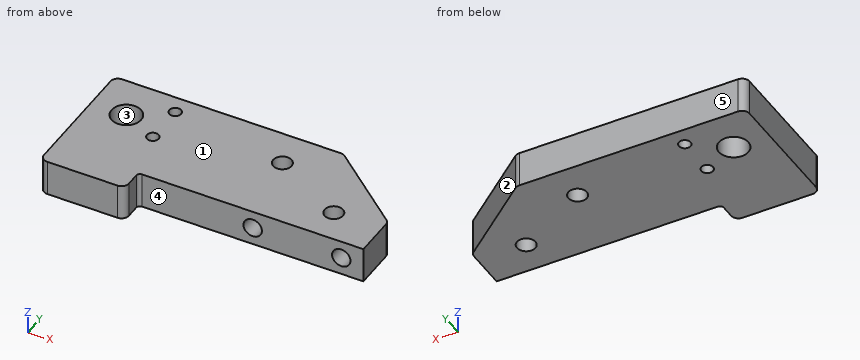
```python
from build123d import *

# Parameters (mm, degrees)
BOSS_EXTRUDE1_DEPTH             = 4.826
M3X0_5_TAPPED_HOLE1_D           = 2.5
TAP_DRILL_FOR_M3X0_5_TAP1_D     = 2.5
TAP_DRILL_FOR_M3X0_5_TAP1_DEPTH = 5
TAP_DRILL_FOR_M3X0_5_TAP1_TIP   = 0.751075774
M3X0_5_TAPPED_HOLE2_D           = 2.5
SKETCH1_3_R                     = 2
BOSS_EXTRUDE2_DEPTH             = 4.826
FILLET1_R                       = 1
M2_TAPPED_HOLES_D               = 1.6
FILLET2_R                       = 0.5


with BuildPart() as part:
    # Sketch1 → Boss-Extrude1 (new body)
    with BuildSketch(Plane.XY):
        Polygon((11, 0), (0, 0), (-11, 0), (-11, 15), (0, 15), (11, 6), align=None)
    extrude(amount=BOSS_EXTRUDE1_DEPTH)

    # M3x0.5 Tapped Hole1 (through all)
    with Locations(Plane.XY.offset(4.826)):
        with Locations((-5.5, 10)):
            Hole(M3X0_5_TAPPED_HOLE1_D / 2)

    # Tap Drill for M3x0.5 Tap1
    with Locations(Plane(origin=(-4, 0, 2.413), x_dir=(-1, 0, 0), z_dir=(0, -1, 0))):
        with Locations((0, 0), (-12, 0)):
            Hole(TAP_DRILL_FOR_M3X0_5_TAP1_D / 2, depth=TAP_DRILL_FOR_M3X0_5_TAP1_DEPTH)
            with Locations((0, 0, -(TAP_DRILL_FOR_M3X0_5_TAP1_DEPTH + TAP_DRILL_FOR_M3X0_5_TAP1_TIP / 2))):  # 118° drill point
                Cone(0, TAP_DRILL_FOR_M3X0_5_TAP1_D / 2, TAP_DRILL_FOR_M3X0_5_TAP1_TIP, mode=Mode.SUBTRACT)

    # M3x0.5 Tapped Hole2 (through all)
    with Locations(Plane(origin=(4.5, 4.5, 4.826), x_dir=(1, 0, 0), z_dir=(0, 0, 1))):
        with Locations((0, 0)):
            Hole(M3X0_5_TAPPED_HOLE2_D / 2)

    # Sketch1<3> → Boss-Extrude2 (add)
    with BuildSketch(Plane.XY):
        Polygon((-19.5, 0), (-11, 0), (-11, 15), (-19.5, 15), (-31, 15), (-31, -3.3), (-19.5, -3.3), align=None)
        with Locations((-26.2, 9.2)):
            Circle(SKETCH1_3_R, mode=Mode.SUBTRACT)
    extrude(amount=BOSS_EXTRUDE2_DEPTH)

    # Fillet1
    fillet1_edges = [part.edges().sort_by_distance(p)[0] for p in [
        (0, 15, 2.413),
        (11, 6, 2.413),
        (-31, 15, 2.413),
        (-31, -3.3, 2.413),
        (-19.5, -3.3, 2.413),
    ]]
    fillet(fillet1_edges, radius=FILLET1_R)

    # M2 Tapped Holes (through all)
    with Locations(Plane.XY.offset(4.826)):
        with Locations((-21.4, 12.5), (-21.4, 7)):
            Hole(M2_TAPPED_HOLES_D / 2)

    # Fillet2
    fillet2_edges = [part.edges().sort_by_distance(p)[0] for p in [
        (-19.5, 0, 2.413),
    ]]
    fillet(fillet2_edges, radius=FILLET2_R)


solid = part.part
```
Check sheet for the modelled part. Datum: model origin and axes. Units: mm. Face numbers are marked on the shaded views. A direction names the side the tool comes from. Coordinates: 2 decimals unless noted, no trailing zeros. Write each loop counter-clockwise with the first axis right and the second up, starting at its lowest first coordinate (ties: lowest second). Pieces come first, ordered by that corner, then holes. Notation, with made-up numbers: M -1.5,11.25 L 24.5,11.25 A20 cw 24.5,22.25 Z; hole C -4.75,11.5 d8. An arc over 180 degrees is marked long. Use one line per item in the form item = value.
Item 1: Release check for a two-part mould opening along X. For the marked faces 1, 2 and 3 record: pulls with the +X half, pulls with the -X half, needs draft (parallel to the pull), parting line crosses it, or undercut.
Answer below:
face_1 = needs draft
face_2 = pulls with the +X half
face_3 = undercut
Item 2: Sectioned sample at A-A, the plane x = -26.2. Record the cut outline in (y, z), and give its area (3 significant figures).
Answer below:
outline = M -3.3,0 L 7.2,0 L 7.2,4.83 L -3.3,4.83 Z; M 11.2,0 L 15,0 L 15,4.83 L 11.2,4.83 Z
area = 69.0 mm^2
Item 3: Sectioned sample at B-B, the plane z = 4.3. Record the cut outline in (x, y), and give its area (3 significant figures).
Answer below:
outline = M -31,-2.3 A1 ccw -30,-3.3 L -20.5,-3.3 A1 ccw -19.5,-2.3 L -19.5,-0.5 A0.5 cw -19,0 L 11,0 L 11,5.53 A1 ccw 10.63,6.3 L 0.28,14.77 A1 ccw -0.36,15 L -30,15 A1 ccw -31,14 Z; hole C -26.2,9.2 d4; hole C -21.4,7 d1.6; hole C -21.4,12.5 d1.6; hole C -5.5,10 d2.5; hole C 4.5,4.5 d2.5
area = 591 mm^2
Item 4: Gauge pin test, flat ends, axial feed: pin 1 Ø3 at (x, y) = (4.5, 4.5) entering from -Z; pin 2 Ø1.3 at (x, y) = (-21.4, 7) entering from +Z; pin 3 Ø2 at (x, z) = (8, 2.413) entering from -Y; pin 4 Ø1.5 at (x, z) = (-4, 2.413) entering from -Y. Record the tip position at first contact, or that the pin passes through.
Answer below:
pin_1 = 0
pin_2 = through
pin_3 = 5.15
pin_4 = 5.3
Item 5: Set-up check for the marked faces 4 and 5: record each of +Z, -Z, +X, -X, +Y, -Y from which the full face is reachable in a straight line by a thin tool's end or side.
Answer below:
face_4 = +Z, -Z, +X, -Y
face_5 = +Z, -Z, +X, -X, +Y
Item 6: Material ranges on L1, parallel to Y at x = -21.4, z = 2.2; L2, parallel to Y at x = -26.2, z = 2.8; L3, parallel to X at y = 2.5, z = 2.7, recorded low to high. Write a range as from..to.
Answer below:
L1 = -3.3..6.2, 7.8..11.7, 13.3..15
L2 = -3.3..7.2, 11.2..15
L3 = -31..-5.22, -2.78..6.78, 9.22..11
Item 7: Sectioned sample at C-C, the plane y = 8.25. Record the cut outline in (x, z), and give its area (3 significant figures).
Answer below:
outline = M -31,0 L -27.96,0 L -27.96,4.83 L -31,4.83 Z; M -24.44,0 L 8.25,0 L 8.25,4.83 L -24.44,4.83 Z
area = 172 mm^2
Item 8: Sectioned sample at D-D, the plane x = -21. Record the cut outline in (y, z).
Answer below:
outline = M -3.3,0 L 6.31,0 L 6.31,4.83 L -3.3,4.83 Z; M 7.69,0 L 11.81,0 L 11.81,4.83 L 7.69,4.83 Z; M 13.19,0 L 15,0 L 15,4.83 L 13.19,4.83 Z
